Check sheet for the modelled part. Datum: model origin and axes. Units: mm. A direction names the side the tool comes from. Give positions to 0.01 mm unless a question says otherwise; leave off trailing zeros. Order: outer loops, then holes, each group sorted by start corner. A loop starts at its lowest first (then second) coordinate and runs counter-clockwise, first axis right, second up. Notation, with made-up numbers: (-9.75, -28.75) -> (22.25, -28.75) arc R19 cw to (22.25, 6.25) -> close; hole circle Ø10 at (80.25, 85.5). An arc over 180 degrees is marked (long way). One line per question, with ' | ' between items.
```python
from build123d import *

# Parameters (mm, degrees)
F0_R     = 10.71035
F1_DEPTH = 50.8
F3_DEPTH = 25.4


with BuildPart() as f1:
    # F0 (on Front) → F1 (new body)
    with BuildSketch(Plane.XZ):
        Circle(F0_R)
    extrude(amount=F1_DEPTH)

    # F2 (on face) → F3 (join)
    with BuildSketch(Plane.XZ.offset(50.8)):
        Polygon((20.402551, -35.032415), (40.540237, 0.15292), (20.137686, 35.185335), (-20.402551, 35.032415), (-40.540237, -0.15292), (-20.137686, -35.185335), align=None)
    extrude(amount=F3_DEPTH)

    # F4: F1 across plane


with BuildPart() as f1_1:
    add(f1.part)
    add(f1.part.mirror(Plane.XZ))


solid = f1_1.part
```
Q1. Section check A-A (x = -14). Enter the section's corners in (y, z), and give its area (3 significant figures).
Result sheet:
outline: (-76.2, -35.16) -> (-50.8, -35.16) -> (-50.8, 35.06) -> (-76.2, 35.06) -> close; (50.8, -35.16) -> (76.2, -35.16) -> (76.2, 35.06) -> (50.8, 35.06) -> close | area: 3,570 mm2
Q2. Section check C-C (x = 0). Enter the section's corners in (y, z), and give its area (3 significant figures).
Result sheet:
outline: (-76.2, -35.11) -> (-50.8, -35.11) -> (-50.8, -10.71) -> (50.8, -10.71) -> (50.8, -35.11) -> (76.2, -35.11) -> (76.2, 35.11) -> (50.8, 35.11) -> (50.8, 10.71) -> (-50.8, 10.71) -> (-50.8, 35.11) -> (-76.2, 35.11) -> close | area: 5,740 mm2
Q3. Depth check by flat-ended pin: pin 1 Ø6 at (x, y) = (10.5, -54) entering from -Z; pin 2 Ø4 at (x, y) = (6, 19) entering from -Z; pin 3 Ø8 at (y, z) = (60.5, -20.5) entering from +X. Enter the tip coordinate at first touch or a pass-through.
Result sheet:
pin 1: stops at z = -35.08 | pin 2: stops at z = -9.94 | pin 3: stops at x = 31.01
Q4. Access from +Z, -Z, +X, -X, +Y, -Y to the whole of each face (thin tool, end or side, straight path). Record for faces 1 (the face through (8.4, -50.8, -7.3)), 2 (the face through (-1, -76.2, 0)).
Result sheet:
face 1: none | face 2: +Z, -Z, +X, -X, -Y
Q5. Thickness scan on line 1 (Y direction, x = -36.5, z = -3); line 2 (Z direction, x = -13.5, y = -55.5); line 3 (Z direction, x = 11.5, y = -57.5). Record the ranges inside material, lowest first.
Result sheet:
line 1: y = -76.2 to -50.8, 50.8 to 76.2 | line 2: z = -35.16 to 35.06 | line 3: z = -35.07 to 35.15
Q6. Section check B-B (z = -28). Enter the section's corners in (x, y).
Result sheet:
outline: (-24.32, -76.2) -> (24.43, -76.2) -> (24.43, -50.8) -> (-24.32, -50.8) -> close; (-24.32, 50.8) -> (24.43, 50.8) -> (24.43, 76.2) -> (-24.32, 76.2) -> close
Q7. Mould release check, pull along Y, two halves, no side actions. Record for faces 3 (the face through (-1, 76.2, 0)), 4 (the face through (8.4, 50.8, -7.3)), 5 (the face through (-30.482, -63.322, -17.424)): pulls with the +Y half, pulls with the -Y half, needs draft (parallel to the pull), parting line crosses it, or undercut.
Result sheet:
face 3: pulls with the +Y half | face 4: undercut | face 5: needs draft
Q8. Section check D-D (y = -58). Enter the section's corners in (x, z), and give its area (3 significant figures).
Result sheet:
outline: (-40.54, -0.15) -> (-20.14, -35.19) -> (20.4, -35.03) -> (40.54, 0.15) -> (20.14, 35.19) -> (-20.4, 35.03) -> close | area: 4,270 mm2
